Could you check a few things on this model? Use its own coordinates, in mm. A direction names the side the tool comes from. Coordinates: 2 decimals unless noted, no trailing zeros. Loops run counter-clockwise (first coordinate to the right, second up) from the corner with the lowest first, then second, coordinate; pieces in that order, holes last.
1) Thinking about a two-plate mould opening in Z: for faces 4 (the face through (7, 29.838, 18)), 5 (the face through (14.15, 6.838, -0.07)), 6 (the face through (19.524, 30.824, -4.336)), which applies, released by +Z, released by -Z, zero draft, split by the parting line, or undercut?
2) For faces 1 (the face through (14.15, 9.838, 0.07)), 2 (the face through (-13.43, 31.838, 8.98)), 3 (the face through (15.62, -4.01, -3.47)), which set-ups out of +Z, -Z, +X, -X, +Y, -Y let a thin tool reach every point of the face, with its end or its side?
3) Imagine slicing it at A-A on z = 0. Please give me the cut outline in (x, y), plus the area to 3 significant figures.
4) Imagine slicing it at B-B on x = 0. Please give me the cut outline in (y, z).
5) Will these pins go through, and if not, where does the flat tip stop? P1, Ø12, axis at x = -11, y = -7, coming from the +Z side; P2, Ø8, axis at x = -8, y = -4, coming from the -Z side; P3, Ø16, axis at x = -2, z = 2, coming from the +Y side; P4, Ø1, axis at x = 4, y = 12.5, coming from the +Z side.
6) If I drill on line 1 along X through (y, z) = (8.15, 0); line 2 along X through (y, z) = (-2.75, 0); line 3 along Z through (x, y) = (5, 24), over which ranges is the centre line in solid material (lowest first)?
7) Imagine slicing it at C-C on y = 21. Please give me the cut outline in (x, z).
```python
from build123d import *


with BuildPart() as part:
    # Esquisse1 → Révolution1 (revolve)
    with BuildSketch(Plane.XY, mode=Mode.PRIVATE) as r_volution1_sk:
        Polygon((-16, -15.162162162), (-16, 6.837837838), (-14, 6.837837838), (-14, 9.837837838), (-16, 9.837837838), (-16, 31.837837838), (-20, 31.837837838), (-20, 29.837837838), (-19, 29.837837838), (-19, -15.162162162), align=None)
    revolve(r_volution1_sk.sketch.rotate(Axis((0, 35.189189189, 0), (0, -1, 0)), 270), axis=Axis((0, 35.189189189, 0), (0, -1, 0)))


solid = part.part
```
Filled in:
1. face 4: zero draft
1. face 5: undercut
1. face 6: split by the parting line
2. face 1: +Y
2. face 2: +Z, -Z, +X, -X, +Y
2. face 3: -Y
3. outline: (-20, 29.84) - (-19, 29.84) - (-19, -15.16) - (-16, -15.16) - (-16, 6.84) - (-14, 6.84) - (-14, 9.84) - (-16, 9.84) - (-16, 31.84) - (-20, 31.84) - close; (14, 6.84) - (16, 6.84) - (16, -15.16) - (19, -15.16) - (19, 29.84) - (20, 29.84) - (20, 31.84) - (16, 31.84) - (16, 9.84) - (14, 9.84) - close
3. area: 298 mm2
4. outline: (-15.16, -19) - (29.84, -19) - (29.84, -20) - (31.84, -20) - (31.84, -16) - (9.84, -16) - (9.84, -14) - (6.84, -14) - (6.84, -16) - (-15.16, -16) - close; (-15.16, 16) - (6.84, 16) - (6.84, 14) - (9.84, 14) - (9.84, 16) - (31.84, 16) - (31.84, 20) - (29.84, 20) - (29.84, 19) - (-15.16, 19) - close
5. P1: stops at z = 18.33
5. P2: stops at z = -18.57
5. P3: passes through
5. P4: stops at z = 18.67
6. line 1: x = -19 to -14, 14 to 19
6. line 2: x = -19 to -16, 16 to 19
6. line 3: z = -18.33 to -15.2, 15.2 to 18.33
7. outline: circle Ø38 at (0, 0); hole circle Ø32 at (0, 0)
